from build123d import *

# Parameters (mm, degrees)
SKETCH1_R      = 1.6
SKETCH1_R_2    = 1.1
SKETCH1_W      = 13.25
SKETCH1_H      = 9.5
EXTRUDE1_DEPTH = 3
FILLET_1_R     = 2


with BuildPart() as part:
    # Sketch1 → Extrude1 (new body)
    with BuildSketch(Plane(origin=(0, 0, 0), x_dir=(1, 0, 0), z_dir=(0, 1, 0))):
        Polygon((30.90824759, 164.13031435), (131.90824759, 164.13031435), (140.90824759, 173.13031435), (140.90824759, 195.63031435), (95.90824759, 195.63031435), (95.90824759, 184.63031435), (87.90824759, 184.63031435), (87.90824759, 195.63031435), (48.90824759, 195.63031435), (48.90824759, 184.63031435), (40.90824759, 184.63031435), (40.90824759, 195.63031435), (30.90824759, 195.63031435), align=None)
        with Locations(Location((131.40824759, 190.63031435, 0), (0, 0, 270))):
            Circle(SKETCH1_R, mode=Mode.SUBTRACT)
        with Locations(Location((99.40824759, 190.63031435, 0), (0, 0, 270))):
            Circle(SKETCH1_R, mode=Mode.SUBTRACT)
        with Locations(Location((82.40824759, 190.63031435, 0), (0, 0, 270))):
            Circle(SKETCH1_R, mode=Mode.SUBTRACT)
        with Locations(Location((54.40824759, 190.63031435, 0), (0, 0, 270))):
            Circle(SKETCH1_R, mode=Mode.SUBTRACT)
        with Locations(Location((35.90824759, 190.63031435, 0), (0, 0, 270))):
            Circle(SKETCH1_R, mode=Mode.SUBTRACT)
        with Locations(Location((112.15824759, 167.63031435, 0), (0, 0, 270))):
            Circle(SKETCH1_R_2, mode=Mode.SUBTRACT)
        with Locations(Location((95.15824759, 167.63031435, 0), (0, 0, 270))):
            Circle(SKETCH1_R_2, mode=Mode.SUBTRACT)
        with Locations(Location((59.65824759, 167.63031435, 0), (0, 0, 270))):
            Circle(SKETCH1_R_2, mode=Mode.SUBTRACT)
        with Locations(Location((42.65824759, 167.63031435, 0), (0, 0, 270))):
            Circle(SKETCH1_R_2, mode=Mode.SUBTRACT)
        with Locations(Location((136.90824759, 176.13031435, 0), (0, 0, 270))):
            Circle(SKETCH1_R_2, mode=Mode.SUBTRACT)
        with Locations(Location((136.90824759, 182.13031435, 0), (0, 0, 270))):
            Circle(SKETCH1_R_2, mode=Mode.SUBTRACT)
        with Locations((119.28324759, 174.88031435)):
            Rectangle(SKETCH1_W, SKETCH1_H, mode=Mode.SUBTRACT)
        with Locations((94.03324759, 174.88031435)):
            Rectangle(SKETCH1_W, SKETCH1_H, mode=Mode.SUBTRACT)
        with Locations((43.53324759, 174.88031435)):
            Rectangle(SKETCH1_W, SKETCH1_H, mode=Mode.SUBTRACT)
        with Locations((68.78324759, 174.88031435)):
            Rectangle(SKETCH1_W, SKETCH1_H, mode=Mode.SUBTRACT)
    extrude(amount=EXTRUDE1_DEPTH)

    # 圆角1
    fillet_1_edges = [part.edges().sort_by_distance(p)[0] for p in [
        (36.90824759, 1.5, -170.13031435),
        (50.15824759, 1.5, -170.13031435),
        (50.15824759, 1.5, -179.63031435),
        (36.90824759, 1.5, -179.63031435),
        (62.15824759, 1.5, -170.13031435),
        (75.40824759, 1.5, -170.13031435),
        (75.40824759, 1.5, -179.63031435),
        (62.15824759, 1.5, -179.63031435),
        (40.90824759, 1.5, -184.63031435),
        (48.90824759, 1.5, -184.63031435),
        (87.90824759, 1.5, -184.63031435),
        (95.90824759, 1.5, -184.63031435),
        (112.65824759, 1.5, -179.63031435),
        (112.65824759, 1.5, -170.13031435),
        (125.90824759, 1.5, -170.13031435),
        (125.90824759, 1.5, -179.63031435),
        (87.40824759, 1.5, -179.63031435),
        (87.40824759, 1.5, -170.13031435),
        (100.65824759, 1.5, -170.13031435),
        (100.65824759, 1.5, -179.63031435),
    ]]
    fillet(fillet_1_edges, radius=FILLET_1_R)


solid = part.part
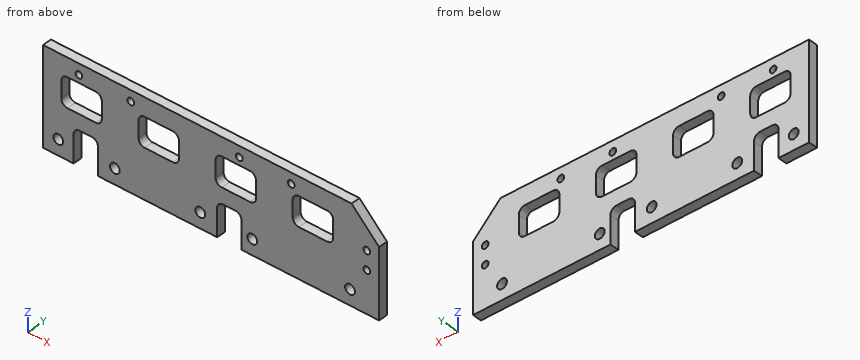
Check sheet for the modelled part. Datum: model origin and axes. Units: mm. Give positions to 0.01 mm unless a question says otherwise; leave off trailing zeros. Loops run counter-clockwise (first coordinate to the right, second up) from the corner with the lowest first, then second, coordinate; pieces in that order, holes last. Notation, with made-up numbers: M -1,76 L 8,76 A31 ccw 8,108 Z; hole C -39.75,-15 d7. An arc over 180 degrees is marked long. Answer as a JSON object with one key per item and string values. Group by question number.
Q1. Material ranges on line 1 along X through (y, z) = (1.1, -188); line 2 along X through (y, z) = (0.4, -174); line 3 along X through (y, z) = (1.65, -185.5), recorded low to high. Write a range as [from, to].
Q2. Cross-section at D-D on x = 134.5. Record the cut outline in (y, z), then the cut area to 3 significant figures.
Q3. Cross-section at B-B on z = -190. Give the number of separate pieces and of enclosed holes in the cut face, then the cut area to 3 significant figures.
Q4. Go/stop test with flat-tipped pins: P1, Ø0.9, axis at x = 43.5, y = 1.5, coming from the -Z side; P2, Ø1.5, axis at x = 47, y = 2.5, coming from the -Z side. Record where each tip stops, or that it passes through.
Q5. Cross-section at A-A on x = 70. Record the cut outline in (y, z).
Evaluation:
{
 "1": {"line 1": "x = [30.91, 40.91], [48.91, 87.91], [95.91, 140.91]", "line 2": "x = [30.91, 36.91], [50.16, 62.16], [75.41, 87.41], [100.66, 112.66], [125.91, 140.91]", "line 3": "x = [30.91, 41.26], [48.56, 88.26], [95.56, 140.91]"},
 "2": {"outline": "M 0,-195.63 L 3,-195.63 L 3,-166.72 L 0,-166.72 Z", "area": "86.7 mm2"},
 "3": {"separate pieces": "8", "enclosed holes": "0", "area": "238 mm2"},
 "4": {"P1": "stops at z = -184.63", "P2": "stops at z = -184.82"},
 "5": {"outline": "M 0,-195.63 L 3,-195.63 L 3,-179.63 L 0,-179.63 Z; M 0,-170.13 L 3,-170.13 L 3,-164.13 L 0,-164.13 Z"}
}
